Autodesk Inventor part; units mm, degrees
ref_plane "Work Plane1" through (4, 0, 0) normal (0, 0.5, 0.866) x (1, 0, 0)
ref_plane "YZ Plane" through (0, 0, 0) normal (1, 0, 0) x (0, 1, 0)
ref_plane "XZ Plane" through (0, 0, 0) normal (0, 1, 0) x (-1, 0, 0)
sketch "Skizze1" plane through (0, 0, 0) normal (0, 0, 1) x (1, 0, 0)
  line L0 (0, 0) -> (4.1667, 0)
  line L1 (8, 1.4434) -> (8, 2.5)
  line L2 (8, 2.5) -> (0, 2.5)
  line L3 (8, 1.4434) -> (5, 1.4434)
  line L4 (5, 1.4434) -> (4.1667, 0)
  line L5 (0, -0.5) -> (0, 3)
  line L6 (0, 2.5) -> (0, 0)
  dimension "d0" = 3
  dimension "d1" = 60
  dimension "d2" = 5
  dimension "d3" = 2.8868
  dimension "d5" = 8
revolve "Körper" add sketch "Skizze1" angle 360 about axis through (0, 0, 0) along (1, 0, 0)
chamfer "Fase1" distance 0.4908 angle 45 1 edges at (8, -2.5, 0) measured on face at (8, 2.1096, -0.3146)
sketch "Skizze2" plane through (8, 0, 0) normal (1, 0, 0) x (0, 0, -1)
  circle A0 centre (0, 0) radius 1.4434
  line L0 (-0.7217, 1.25) -> (0.7217, 1.25)
  line L1 (0.7217, 1.25) -> (1.4434, 0)
  line L2 (1.4434, 0) -> (0.7217, -1.25)
  line L3 (0.7217, -1.25) -> (-0.7217, -1.25)
  line L4 (-0.7217, -1.25) -> (-1.4434, 0)
  line L5 (-1.4434, 0) -> (-0.7217, 1.25)
extrude "Loch" add sketch "Skizze2" against normal up to next contours L1 A0 | A0 L2 | L0 A0 | A0 L3 | L5 A0 | A0 L4
thread "Gewinde"
chamfer "Fase2" distance 0.4908 angle 45 1 edges at (0, -2.5, 0) measured on face at (2.5031, 2.4676, -0.401)
ref_plane "Work Plane1" through (4, 0, 0) normal (0, 0.5, 0.866) x (1, 0, 0)
equation "\"d0\" = INTI"
equation "\"d2\" = NND"
equation "\"d3\" = 1.1547 * SW"
equation "\"d5\" = NLG"
equation "\"d7\" = -0.5 * GD1 + 0.5 * NND"
equation "\"d8\" = FAWI"
equation "\"d29\" = -0.5 * GD1 + 0.5 * NND"
equation "\"d11\" = NLG"
equation "\"d13\" = -0.5 * GD1 + 0.5 * NND"
equation "\"d14\" = FAWI"
equation "\"d30\" = -0.5 * GD1 + 0.5 * NND"
equation "\"NND\" = 5"
equation "\"NLG\" = 8"
equation "\"INTI\" = 3"
equation "\"FAWI\" = 45deg"
equation "\"SW\" = 2.5"
equation "\"GD1\" = THREADDIA - 1.2269 * PTC"
equation "\"FAWI1\" = 45deg"
equation "\"GUL\" = 0.61345 * PTC"
equation "\"SPD\" = 3.5"
equation "\"SEWI\" = 90deg"
equation "\"TOA\" = 30deg"
equation "\"THREADDIA\" = 5"
equation "\"PTC\" = 0.8"
equation "\"GAL\" = 0.61345 * PTC"
equation "\"E0\" = 1.155 * SW"
properties part number "ISO 4026 - M5 x 8" material "Edelstahl, 440C"
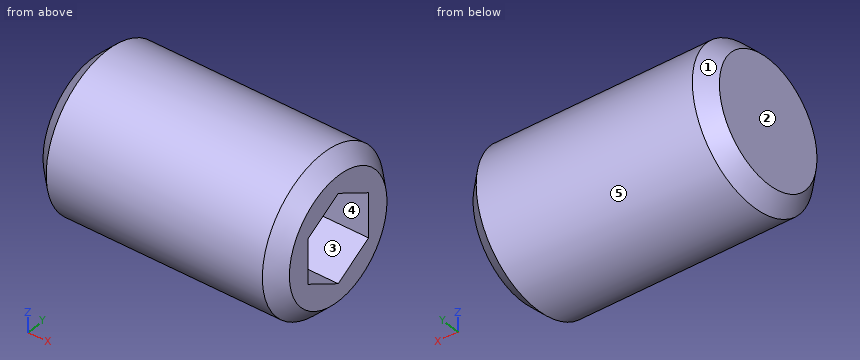
Input: part model. Units: mm. Frame: model coordinates. Face numbers are marked on the shaded views. A direction names the side the tool comes from. Give positions to 0.01 mm unless a question says otherwise; leave off trailing zeros. Loops run counter-clockwise (first coordinate to the right, second up) from the corner with the lowest first, then second, coordinate; pieces in that order, holes last. Notation, with made-up numbers: (-26.75, 39) -> (3.25, 39) arc R29 cw to (3.25, 72) -> close; hole circle Ø5 at (-2, 75). An arc over 180 degrees is marked (long way). Answer as a JSON object with one key per item and string values. Group by question number.
Item 1: Cut plane B-B, the plane x = 3.25. Return the cut outline in (y, z), and give its area (3 significant figures).
Item 2: Reachability of the marked faces 4 and 5 from +Z, -Z, +X, -X, +Y, -Y: full face, straight path, thin tool, end or side. Return the list, or none.
Item 3: Line query: probe 1 along Y at (x, z) = (2, 0.1); probe 2 along Y at (x, z) = (5.5, -0.1); probe 3 along Y at (x, z) = (6.5, 1.1) (3 decimals). Output: solid intervals per line, ascending.
Item 4: Pull-direction query (Y, two-part tool) for the marked faces 1, 2 and 3; classes: released by +Y, released by -Y, zero draft, split by the parting line, or undercut.
Item 5: Cut plane A-A, the plane x = 7. Return the cut outline in (y, z).
Checks:
{
 "1": {"outline": "circle Ø5 at (0, 0)", "area": "19.6 mm²"},
 "2": {"face 4": "+X", "face 5": "+X, -X"},
 "3": {"probe 1": "y = -2.5 to 2.5", "probe 2": "y = -2.5 to -1.25, 1.25 to 2.5", "probe 3": "y = -2.245 to -0.595, 0.595 to 2.245"},
 "4": {"face 1": "split by the parting line", "face 2": "zero draft", "face 3": "undercut"},
 "5": {"outline": "circle Ø5 at (0, 0); hole (-1.25, -0.72) -> (0, -1.44) -> (1.25, -0.72) -> (1.25, 0.72) -> (0, 1.44) -> (-1.25, 0.72) -> close"}
}
